CAD build for the part. Positions are in the model's coordinates, mm. A direction names the side the tool comes from. Round coordinates to 2 decimals unless told otherwise and drop trailing zeros. Use a Markdown table: item, result. Add a question column.
(1) Two-plate mould, pull along Y, no slides. Class faces 6 (the face through (1, 1, -1)), 7 (the face through (-65.359, -45.297, 2.465)), 8 (the face through (62, -44, 2)): released by +Y, released by -Y, zero draft, split by the parting line, or undercut.
(2) Wall check: L1, parallel to Y at x = 62.5, z = 0.55; L2, parallel to Y at x = -62.5, z = 4.45; L3, parallel to X at y = 42, z = 2.3. Give the ranges that are in metal, low to high.
(3) Which spindle directions (+Z, -Z, +X, -X, +Y, -Y) get a long thin tool onto all of the face, cutting with end or side? Do faces 1 (the face through (-59.654, -39.689, -0.254)), 2 (the face through (-59.689, 39.654, -0.254)), 3 (the face through (59.654, 39.689, -0.254)), 4 (the face through (59.689, -39.654, -0.254)), 5 (the face through (60, 43, 3)). Say none if no direction does.
(4) Flat gauge pins, fed straight in: P1, Ø3, axis at x = 62.5, y = 42.5, coming from the +Z side; P2, Ø3, axis at x = -62.5, y = -42.5, coming from the +Z side; P3, Ø4.5, axis at x = -62.5, y = 42.5, coming from the -Z side. Where does each tip first touch, or does it go through?
from build123d import *

# Parameters (mm, degrees)
SKETCH2_R           = 1.25
BOSS_EXTRUDE1_DEPTH = 2
SKETCH3_R           = 2.55
BOSS_EXTRUDE2_DEPTH = 3
BOSS_EXTRUDE3_START = 3
BOSS_EXTRUDE3_DEPTH = 3
CHAMFER1_SIZE       = 0.5
CHAMFER2_SIZE       = 1.5


with BuildPart() as part:
    # Sketch2 → Boss-Extrude1 (new body)
    with BuildSketch(Plane.XY):
        with BuildLine():
            Line((66.5, -42.5), (66.5, 42.5))
            ThreePointArc((66.5, 42.5), (65.328427125, 45.328427125), (62.5, 46.5))
            Line((62.5, 46.5), (-62.5, 46.5))
            ThreePointArc((-62.5, 46.5), (-65.328427125, 45.328427125), (-66.5, 42.5))
            Line((-66.5, 42.5), (-66.5, -42.5))
            ThreePointArc((-66.5, -42.5), (-65.328427125, -45.328427125), (-62.5, -46.5))
            Line((-62.5, -46.5), (62.5, -46.5))
            ThreePointArc((62.5, -46.5), (65.328427125, -45.328427125), (66.5, -42.5))
        make_face()
        with Locations((-62.5, 42.5)):
            Circle(SKETCH2_R, mode=Mode.SUBTRACT)
        with Locations((62.5, 42.5)):
            Circle(SKETCH2_R, mode=Mode.SUBTRACT)
        with Locations((-62.5, -42.5)):
            Circle(SKETCH2_R, mode=Mode.SUBTRACT)
        with Locations((62.5, -42.5)):
            Circle(SKETCH2_R, mode=Mode.SUBTRACT)
        with BuildLine():
            Line((-62.5, -36.843145751), (-62.5, 36.843145751))
            ThreePointArc((-62.5, 36.843145751), (-62.132993162, 37.997846289), (-61.166666667, 38.728763834))
            ThreePointArc((-61.166666667, 38.728763834), (-59.671572875, 39.671572875), (-58.728763834, 41.166666667))
            ThreePointArc((-58.728763834, 41.166666667), (-57.997846289, 42.132993162), (-56.843145751, 42.5))
            Line((-56.843145751, 42.5), (56.843145751, 42.5))
            ThreePointArc((56.843145751, 42.5), (57.997846289, 42.132993162), (58.728763834, 41.166666667))
            ThreePointArc((58.728763834, 41.166666667), (59.671572875, 39.671572875), (61.166666667, 38.728763834))
            ThreePointArc((61.166666667, 38.728763834), (62.132993162, 37.997846289), (62.5, 36.843145751))
            Line((62.5, 36.843145751), (62.5, -36.843145751))
            ThreePointArc((62.5, -36.843145751), (62.132993162, -37.997846289), (61.166666667, -38.728763834))
            ThreePointArc((61.166666667, -38.728763834), (59.671572875, -39.671572875), (58.728763834, -41.166666667))
            ThreePointArc((58.728763834, -41.166666667), (57.997846289, -42.132993162), (56.843145751, -42.5))
            Line((56.843145751, -42.5), (-56.843145751, -42.5))
            ThreePointArc((-56.843145751, -42.5), (-57.997846289, -42.132993162), (-58.728763834, -41.166666667))
            ThreePointArc((-58.728763834, -41.166666667), (-59.671572875, -39.671572875), (-61.166666667, -38.728763834))
            ThreePointArc((-61.166666667, -38.728763834), (-62.132993162, -37.997846289), (-62.5, -36.843145751))
        make_face(mode=Mode.SUBTRACT)
    extrude(amount=BOSS_EXTRUDE1_DEPTH)

    # Sketch3 → Boss-Extrude2 (add)
    with BuildSketch(Plane.XY.offset(2)):
        with BuildLine():
            Line((66.5, -42.5), (66.5, 42.5))
            ThreePointArc((66.5, 42.5), (65.328427125, 45.328427125), (62.5, 46.5))
            Line((62.5, 46.5), (-62.5, 46.5))
            ThreePointArc((-62.5, 46.5), (-65.328427125, 45.328427125), (-66.5, 42.5))
            Line((-66.5, 42.5), (-66.5, -42.5))
            ThreePointArc((-66.5, -42.5), (-65.328427125, -45.328427125), (-62.5, -46.5))
            Line((-62.5, -46.5), (62.5, -46.5))
            ThreePointArc((62.5, -46.5), (65.328427125, -45.328427125), (66.5, -42.5))
        make_face()
        with Locations((-62.5, 42.5)):
            Circle(SKETCH3_R, mode=Mode.SUBTRACT)
        with Locations((62.5, 42.5)):
            Circle(SKETCH3_R, mode=Mode.SUBTRACT)
        with Locations((62.5, -42.5)):
            Circle(SKETCH3_R, mode=Mode.SUBTRACT)
        with Locations((-62.5, -42.5)):
            Circle(SKETCH3_R, mode=Mode.SUBTRACT)
    extrude(amount=BOSS_EXTRUDE2_DEPTH)

    # Sketch4 → Boss-Extrude3 (add)
    with BuildSketch(Plane(origin=(0, 0, 2), x_dir=(-1, 0, 0), z_dir=(0, 0, -1)).offset(BOSS_EXTRUDE3_START)):
        with BuildLine():
            Line((62.5, -36.843145751), (62.5, 36.843145751))
            ThreePointArc((62.5, 36.843145751), (62.132993162, 37.997846289), (61.166666667, 38.728763834))
            ThreePointArc((61.166666667, 38.728763834), (59.671572875, 39.671572875), (58.728763834, 41.166666667))
            ThreePointArc((58.728763834, 41.166666667), (57.997846289, 42.132993162), (56.843145751, 42.5))
            Line((56.843145751, 42.5), (-56.843145751, 42.5))
            ThreePointArc((-56.843145751, 42.5), (-57.997846289, 42.132993162), (-58.728763834, 41.166666667))
            ThreePointArc((-58.728763834, 41.166666667), (-59.671572875, 39.671572875), (-61.166666667, 38.728763834))
            ThreePointArc((-61.166666667, 38.728763834), (-62.132993162, 37.997846289), (-62.5, 36.843145751))
            Line((-62.5, 36.843145751), (-62.5, -36.843145751))
            ThreePointArc((-62.5, -36.843145751), (-62.132993162, -37.997846289), (-61.166666667, -38.728763834))
            ThreePointArc((-61.166666667, -38.728763834), (-59.671572875, -39.671572875), (-58.728763834, -41.166666667))
            ThreePointArc((-58.728763834, -41.166666667), (-57.997846289, -42.132993162), (-56.843145751, -42.5))
            Line((-56.843145751, -42.5), (56.843145751, -42.5))
            ThreePointArc((56.843145751, -42.5), (57.997846289, -42.132993162), (58.728763834, -41.166666667))
            ThreePointArc((58.728763834, -41.166666667), (59.671572875, -39.671572875), (61.166666667, -38.728763834))
            ThreePointArc((61.166666667, -38.728763834), (62.132993162, -37.997846289), (62.5, -36.843145751))
        make_face()
    extrude(amount=-BOSS_EXTRUDE3_DEPTH)

    # Chamfer1
    chamfer1_edges = [part.edges().sort_by_distance(p)[0] for p in [
        (-59.671572875, -39.671572875, -1),
        (-62.132993162, -37.997846289, -1),
        (-62.5, 0, -1),
        (-62.132993162, 37.997846289, -1),
        (-59.671572875, 39.671572875, -1),
        (-57.997846289, 42.132993162, -1),
        (0, 42.5, -1),
        (57.997846289, 42.132993162, -1),
        (59.671572875, 39.671572875, -1),
        (62.132993162, 37.997846289, -1),
        (62.5, 0, -1),
        (62.132993162, -37.997846289, -1),
        (59.671572875, -39.671572875, -1),
        (57.997846289, -42.132993162, -1),
        (0, -42.5, -1),
        (-57.997846289, -42.132993162, -1),
    ]]
    chamfer(chamfer1_edges, length=CHAMFER1_SIZE)

    # Chamfer2
    # the kernel refuses this chamfer: 1.5 mm, written as the material it adds along each edge
    with BuildSketch(Plane(origin=(-62.5, -42.5, 2), x_dir=(1, 0, 0), z_dir=(0, -1, 0))) as chamfer2_piece_1_section:
        Polygon((2.55 - CHAMFER2_SIZE, 0), (2.55, CHAMFER2_SIZE), (2.55, 0), align=None)
    chamfer2_piece_1 = revolve(axis=Axis((-62.5, -42.5, 2), (0, 0, 1)), mode=Mode.PRIVATE)
    chamfer2_piece_1 = chamfer2_piece_1 - Plane(origin=(-62.5, -42.5, 2.85349357), x_dir=(1, 0, 0), z_dir=(0, 0, -1)) * Cylinder(1.25, 11, mode=Mode.PRIVATE)
    add(chamfer2_piece_1)


solid = part.part
Return value:
| question | item | result |
|---|---|---|
| 1 | face 6 | zero draft |
| 1 | face 7 | released by -Y |
| 1 | face 8 | undercut |
| 2 | L1 | -46.5 to -43.75, -41.25 to 41.25, 43.75 to 46.5 |
| 2 | L2 | -46.5 to -45.05, -39.95 to 39.95, 45.05 to 46.5 |
| 2 | L3 | -66.5 to -65, -60 to 60, 65 to 66.5 |
| 3 | face 1 | -Z, -X, -Y |
| 3 | face 2 | -Z, -X, +Y |
| 3 | face 3 | -Z, +X, +Y |
| 3 | face 4 | -Z, +X, -Y |
| 3 | face 5 | +Z |
| 4 | P1 | z = 2 |
| 4 | P2 | z = 2.45 |
| 4 | P3 | z = 0 |
